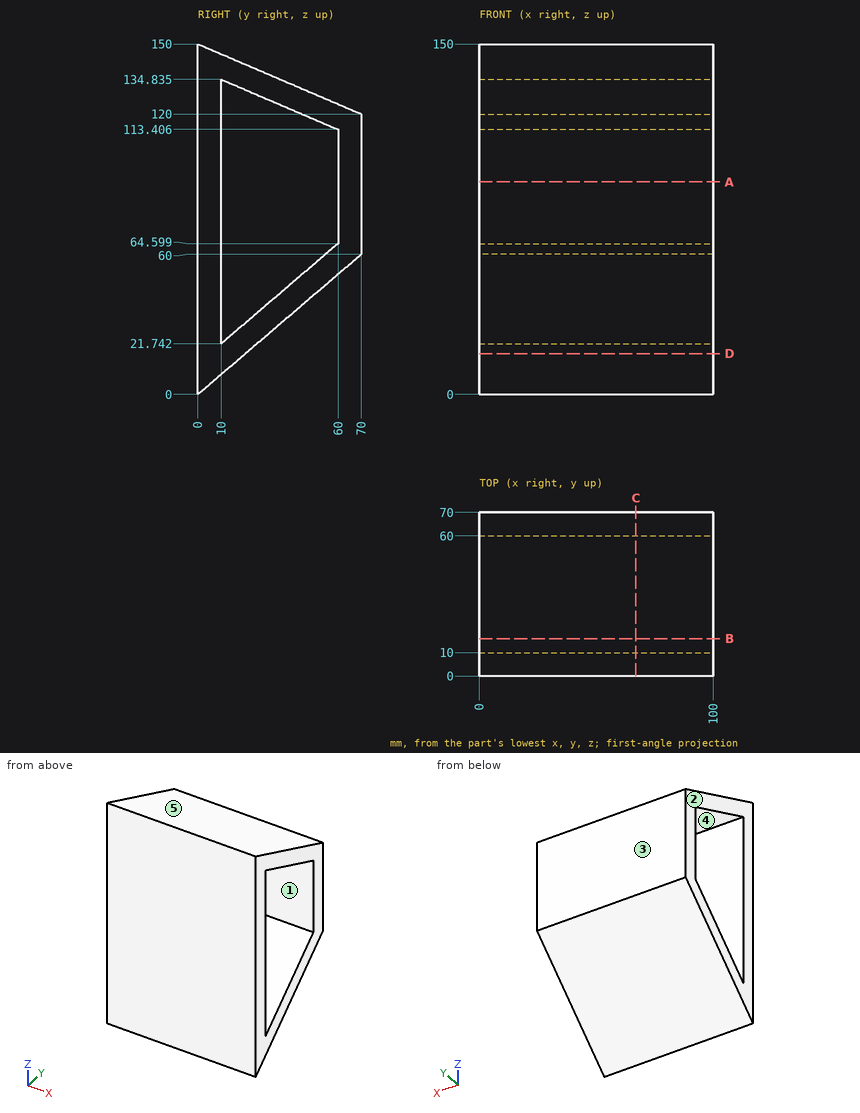
Study the drawing (mm; zero at the part's minimum x, y, z) and answer. A direction names the side the tool comes from. Give positions to 0.01 mm unless a question says otherwise; leave off trailing zeros. Loops run counter-clockwise (first coordinate to the right, second up) from the corner with the lowest first, then second, coordinate; pieces in that order, holes last. Notation, with made-up numbers: (80.25, 2.25) - (99.25, 2.25) arc R21 cw to (99.25, 31.25) - close; hole circle Ø8 at (87, -22.5). An arc over 180 degrees is marked (long way). Answer in a Markdown table with one row per item. Add a question column.
Q1. The part is cut by section A-A (z = 91). Determine the outline of the cut face in (x, y).
Q2. Determine the mould class of the marked faces 3, 4 and 5 for opening direction Z: released by +Z, released by -Z, zero draft, split by the parting line, or undercut.
Q3. The part is cut by section D-D (z = 17.5). Determine the outline of the cut face in (x, y), and give its area (3 significant figures).
Q4. Consider line 1 along Y through (x, z) = (20.5, 97.5); line 2 along Y through (x, z) = (73, 124.5) (1 decimal); line 3 along Z through (x, y) = (61.5, 59) (1 decimal). Determine where each line is inside the solid, lowest interval first.
Q5. A tool of negligible diameter and unlimited length cuts with its end or side. For the marked faces 1 and 2, from which of +Z, -Z, +X, -X, +Y, -Y can it reach the whole face along a straight path? Write none if from no direction.
Q6. The part is cut by section B-B (y = 16). Determine the outline of the cut face in (x, z) (1 decimal), and give its area (4 significant figures).
Q7. The part is cut by section C-C (x = 67). Determine the outline of the cut face in (y, z) (1 decimal).
Q8. Each of these flat-tipped pins is pushed along its axis until it touches: P1, Ø2, axis at x = 19, y = 44.5, coming from the +Z side; P2, Ø4, axis at x = 15, y = 34.5, coming from the -Z side. Where does it stop, or does it pass through?
Solution:
| question | item | result |
|---|---|---|
| 1 | outline | (0, 0) - (100, 0) - (100, 10) - (0, 10) - close; (0, 60) - (100, 60) - (100, 70) - (0, 70) - close |
| 2 | face 3 | zero draft |
| 2 | face 4 | undercut |
| 2 | face 5 | released by +Z |
| 3 | outline | (0, 0) - (100, 0) - (100, 20.42) - (0, 20.42) - close |
| 3 | area | 2,040 mm² |
| 4 | line 1 | y = 0 to 10, 60 to 70 |
| 4 | line 2 | y = 0 to 10, 34.1 to 59.5 |
| 4 | line 3 | z = 50.6 to 63.7, 113.8 to 124.7 |
| 5 | face 1 | +X, -X |
| 5 | face 2 | +Z, -Z, -X, +Y, -Y |
| 6 | outline | (0, 13.7) - (100, 13.7) - (100, 26.9) - (0, 26.9) - close; (0, 132.3) - (100, 132.3) - (100, 143.1) - (0, 143.1) - close |
| 6 | area | 2,405 mm² |
| 7 | outline | (0, 0) - (70, 60) - (70, 120) - (0, 150) - close; hole (10, 21.7) - (60, 64.6) - (60, 113.4) - (10, 134.8) - close |
| 8 | P1 | stops at z = 131.36 |
| 8 | P2 | stops at z = 27.86 |
